Source: CAD feature listing. Evaluate the final solid. Frame: model axes, mm. A direction names the side the tool comes from. Give positions to 0.01 mm unless a question says otherwise; leave off trailing zeros. Loops run counter-clockwise (first coordinate to the right, second up) from the corner with the lowest first, then second, coordinate; pieces in that order, holes last. Notation, with made-up numbers: (47, 39.5) - (80, 39.5) arc R11 cw to (80, 43.5) - close; hole circle Ø3 at (1, 20). An arc over 180 degrees is marked (long way). Put each result on its own line as item: value.
```python
from build123d import *

# Parameters (mm, degrees)
F0_W     = 2
F0_H     = 62
F0_W_2   = 17
F0_W_3   = 14.6
F0_H_2   = 15
F1_DEPTH = 2
F2_DEPTH = 5
F3_DEPTH = 2
F4_SIZE  = 0.5


with BuildPart() as f1:
    # F0 (on Top) → F1 (new body)
    with BuildSketch(Plane.XY):
        with Locations((1, -31)):
            Rectangle(F0_W, F0_H)
        with Locations((10.5, -31)):
            Rectangle(F0_W_2, F0_H)
        with Locations((10.5, -32.5)):
            Rectangle(F0_W_3, F0_H_2, mode=Mode.SUBTRACT)
        with Locations((20, -31)):
            Rectangle(F0_W, F0_H)
        with Locations((10.5, -32.5)):
            Rectangle(F0_W_3, F0_H_2)
    extrude(amount=F1_DEPTH)

    # F0 (on Top) → F2 (join)
    with BuildSketch(Plane.XY):
        with Locations((10.5, -32.5)):
            Rectangle(F0_W_3, F0_H_2)
    extrude(amount=-F2_DEPTH)

    # F0 (on Top) → F3 (join)
    with BuildSketch(Plane.XY):
        with Locations((1, -31)):
            Rectangle(F0_W, F0_H)
        with Locations((20, -31)):
            Rectangle(F0_W, F0_H)
    extrude(amount=-F3_DEPTH)

    # F4
    f4_edges = [f1.edges().sort_by_distance(p)[0] for p in [
        (2, -31, -2),
        (19, -31, -2),
        (3.2, -32.5, -5),
        (17.8, -32.5, -5),
    ]]
    chamfer(f4_edges, length=F4_SIZE)


solid = f1.part
```
1) Pin query (flat end, axial travel): P1, Ø1.6, axis at x = 20, y = -20, coming from the -Z side; P2, Ø1, axis at x = 11, z = -2, coming from the -Y side; P3, Ø4, axis at x = 8, z = -4, coming from the +Y side. Return the tip coordinate at first contact, or that it passes through.
Check result:
P1: z = -2
P2: y = -40
P3: y = -25
2) Section query C-C, the plane y = -35. Output: boundary loops of the cut face in (x, z), plus the area to 4 significant figures.
Check result:
outline: (0, -2) - (1.5, -2) - (2, -1.5) - (2, 0) - (3.2, 0) - (3.2, -4.5) - (3.7, -5) - (17.3, -5) - (17.8, -4.5) - (17.8, 0) - (19, 0) - (19, -1.5) - (19.5, -2) - (21, -2) - (21, 2) - (0, 2) - close
area: 122.5 mm²
3) Material intervals for line 1 along X through (y, z) = (-29, -1.25); line 2 along X through (y, z) = (-5, -1.25); line 3 along Z through (x, y) = (9.5, -44), sorted ascending. Write a range as [from, to].
Check result:
line 1: [0, 2], [3.2, 17.8], [19, 21]
line 2: [0, 2], [19, 21]
line 3: [0, 2]
4) Section query A-A, the plane y = -54. Output: boundary loops of the cut face in (x, z).
Check result:
outline: (0, -2) - (1.5, -2) - (2, -1.5) - (2, 0) - (19, 0) - (19, -1.5) - (19.5, -2) - (21, -2) - (21, 2) - (0, 2) - close
5) Section query B-B, the plane x = 14.5. Output: boundary loops of the cut face in (y, z).
Check result:
outline: (-62, 0) - (-40, 0) - (-40, -5) - (-25, -5) - (-25, 0) - (0, 0) - (0, 2) - (-62, 2) - close
6) Access query for faces 1 (the flat face through (10, -25, -2)), 2 (the flat face through (3.2, -33, -2)), 3 (the flat face through (1, -31, -2)). Directions: +Z, -Z, +X, -X, +Y, -Y. A direction counts if a zero-diameter tool reaches every point of the face in a straight line with its end or side. Return the directions, or none.
Check result:
face 1: -Z, +Y
face 2: -Z, +Y, -Y
face 3: -Z, -X, +Y, -Y
7) Mould query, pull axis X, two halves, no side actions, for faces 4 (the flat face through (10, -24, 0)), 5 (the flat face through (0, -31, 0)), 6 (the flat face through (21, -31, 0)), 7 (the flat face through (10, -32, -5)). Classes: pulls with the +X half, pulls with the -X half, needs draft (parallel to the pull), parting line crosses it, or undercut.
Check result:
face 4: undercut
face 5: pulls with the -X half
face 6: pulls with the +X half
face 7: needs draft
